```python
from build123d import *

# Parameters (mm, degrees)
F0_W       = 225.5908995867
F0_H       = 110.7080131769
F1_DEPTH   = 25.4
F4_D       = 5.08
F4_ON_F3_D = 5.08


with BuildPart() as f1:
    # F0 (on Top) → F1 (new body)
    with BuildSketch(Plane.XY):
        Rectangle(F0_W, F0_H)
    extrude(amount=F1_DEPTH)

    # F4 (through all)
    with Locations(Plane(origin=(0, 0, 0), x_dir=(1, 0, 0), z_dir=(0, 0, -1))):
        with Locations((-89.1955047846, -28.7043005228), (-79.5057713985, -30.0970748067), (-69.9255764484, -28.9903935045), (-68.5980245471, -19.1571637988), (-78.1845897436, -12.9927601665), (-83.154708147, -12.6179577783), (-90.5335843563, -19.003495574), (-89.870005846, -9.1491872445), (-89.4763618708, 0), (-35.4230366647, -30.6281708181), (-42.043376714, -29.9839507788), (-48.6943908036, -22.6104743779), (-53.1893521547, -14.1117144376), (-52.9635697603, -4.1349874809), (-50.1413084567, 1.9611027092), (-28.1036905944, 4.083125852), (-24.3639256805, -3.957584966), (-38.5011509061, 4.5216716826), (-43.8372641802, 4.1484474204), (1.2550167739, -6.3989050686), (-11.9153521955, 11.0068321228), (-4.5298971236, 13.3858900517), (7.5309276581, 11.8151064962), (17.2491893172, 1.2902654707), (15.9244015813, 6.9156782702), (12.3532637954, -5.088057369), (-7.884927094, -10.0290328264), (-23.1754053384, -14.5218074322), (-28.9888959378, -28.0108693987), (-25.011414662, -20.8662394434), (-9.768307209, -16.8593600392), (-10.1366043091, -27.7768112719), (22.8765979409, -40.9418046474), (29.0453359485, -38.6429131031), (36.6399362683, -39.7155433893), (48.0803251266, -38.8907343149), (58.6461164057, -38.6321358383), (9.3805007637, -33.504512161), (0.3481768072, -32.0298522711), (-5.6142956018, -32.4345678091), (38.4009592235, -35.6136150658)):
            Hole(F4_D / 2)

    # F4 on F3 (through all)
    with Locations(Plane(origin=(0, 0, 0), x_dir=(1, 0, 0), z_dir=(0, 0, -1))):
        with Locations((36.813724786, 7.4405698106), (38.6443585157, 0), (38.1508171558, -6.0257110745), (39.7485755384, -13.6793162674), (36.3263972104, -22.3615150899), (37.1932201087, -27.3784212768)):
            Hole(F4_ON_F3_D / 2)

    # F5: F1 across plane


with BuildPart() as f1_1:
    add(f1.part)
    add(f1.part.mirror(Plane.XY))


solid = f1_1.part
```
Verification items for the finished model (mm, model axes). Round coordinates to 2 decimals unless told otherwise and drop trailing zeros.
1. Draft check along X on faces 1 (the flat face through (112.795, -1, 0)), 2 (the flat face through (-2, 55.354, 0)), 3 (the cylindrical face through (-35.09, 28.11, -0.36)), 4 (the cylindrical face through (-67.388, 28.879, -0.356)). Enter one of: +X half, -X half, draft (parallel to the pull), parting line (faces both ways), or undercut.
2. Scan lines: L1, parallel to Y at x = -30, z = 4.5; L2, parallel to Y at x = -81.5, z = 9; L3, parallel to Y at x = -38, z = -16.5. Record each from-to range of solid material in increasing order.
3. Section check A-A on z = 8.5. State how many separate pieces and enclosed holes the cut face has, plus the area to 3 significant figures.
Answer:
1. face 1: +X half
1. face 2: draft
1. face 3: undercut
1. face 4: undercut
2. L1: y = -55.35 to -5.77, -2.39 to 25.68, 30.34 to 55.35
2. L2: y = -55.35 to 10.69, 14.55 to 28.52, 31.67 to 55.35
2. L3: y = -55.35 to -7.01, -2.03 to 55.35
3. separate pieces: 1
3. enclosed holes: 45
3. area: 24,000 mm2
